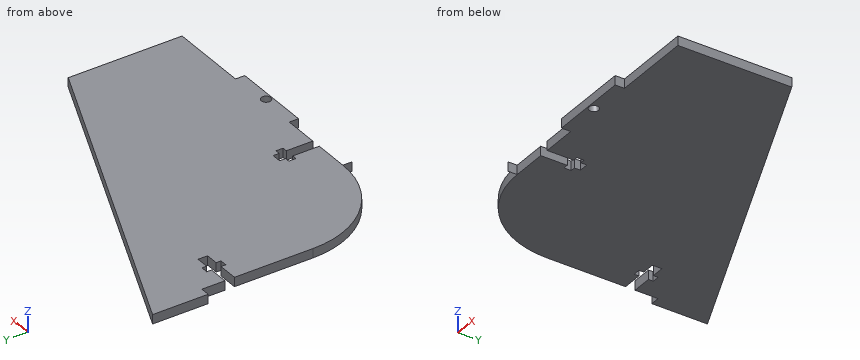
from build123d import *

# Parameters (mm, degrees)
BOSS_EXTRUDE1_DEPTH     = 2.9718
SKETCH3_W               = 2.9718
SKETCH3_H               = 17.78
CUT_EXTRUDE4_DEPTH      = 2.9718
CUT_EXTRUDE4_DEPTH_BACK = 3.9718
SKETCH4_R               = 1.524
CUT_EXTRUDE5_DEPTH      = 2.9718
CUT_EXTRUDE6_DEPTH      = 2.9718
CUT_EXTRUDE7_DEPTH      = 1
CUT_EXTRUDE7_DEPTH_BACK = 2.9718


with BuildPart() as part:
    # Sketch1 → Boss-Extrude1 (new body)
    with BuildSketch(Plane.XY):
        with BuildLine():
            Line((0, 0), (-76.2, 0))
            ThreePointArc((-76.2, 0), (-99.068034345, 9.472249971), (-108.540284316, 32.340284316))
            Line((-108.540284316, 32.340284316), (-108.540284316, 85.680284316))
            Line((-108.540284316, 85.680284316), (0, 39.416788246))
            Line((0, 39.416788246), (0, 0))
        make_face()
    extrude(amount=BOSS_EXTRUDE1_DEPTH)

    # Sketch3 → Cut-Extrude4 (cut, two sides)
    with BuildSketch(Plane.XY.offset(2.9718)) as cut_extrude4_sk:
        Polygon((-25.342092582, 2.9718), (-25.349200788, 0), (0, 0), (0, 2.9718), align=None)
        with BuildLine():
            Line((-76.2, 2.9718), (-76.202051529, 6.5e-08))
            ThreePointArc((-76.202051529, 6.5e-08), (-76.201025765, 1.6e-08), (-76.2, 0))
            Line((-76.2, 0), (-50.8, 0))
            Line((-50.8, 0), (-50.8, 2.9718))
            Line((-50.8, 2.9718), (-76.2, 2.9718))
        make_face()
        with Locations((-107.054384316, 59.010284316)):
            Rectangle(SKETCH3_W, SKETCH3_H)
    extrude(amount=CUT_EXTRUDE4_DEPTH, mode=Mode.SUBTRACT)
    extrude(cut_extrude4_sk.sketch, amount=-CUT_EXTRUDE4_DEPTH_BACK, mode=Mode.SUBTRACT)

    # Sketch4 → Cut-Extrude5 (cut)
    with BuildSketch(Plane.XY.offset(2.9718)):
        with Locations((-38.074600394, 1.794277041)):
            Circle(SKETCH4_R)
    extrude(amount=-CUT_EXTRUDE5_DEPTH, mode=Mode.SUBTRACT)

    # Sketch5 → Cut-Extrude6 (cut)
    with BuildSketch(Plane.XY.offset(2.9718)):
        Polygon((-105.568484316, 60.534284316), (-105.568484316, 59.010284316), (-92.868484316, 59.010284316), (-92.868484316, 60.534284316), (-96.932484316, 60.534284316), (-96.932484316, 62.058284316), (-99.218484316, 62.058284316), (-99.218484316, 60.534284316), align=None)
        Polygon((-92.868484316, 59.010284316), (-105.568484316, 59.010284316), (-105.568484316, 57.486284316), (-99.218484316, 57.486284316), (-99.218484316, 55.962284316), (-96.932484316, 55.962284316), (-96.932484316, 57.486284316), (-92.868484316, 57.486284316), align=None)
        Polygon((-65.024, 2.9718), (-63.5, 2.9718), (-63.5, 15.6718), (-65.024, 15.6718), (-65.024, 13.745923506), (-66.548, 13.745923506), (-66.548, 11.459923506), (-65.024, 11.459923506), align=None)
        Polygon((-63.5, 15.6718), (-63.5, 2.9718), (-61.976, 2.9718), (-61.976, 11.459923506), (-60.452, 11.459923506), (-60.452, 13.745923506), (-61.976, 13.745923506), (-61.976, 15.6718), align=None)
    extrude(amount=-CUT_EXTRUDE6_DEPTH, mode=Mode.SUBTRACT)

    # Sketch6 → Cut-Extrude7 (cut, two sides)
    with BuildSketch(Plane.XY.offset(2.9718)) as cut_extrude7_sk:
        with BuildLine():
            ThreePointArc((-105.568484316, 32.340284316), (-96.967313076, 11.574288587), (-76.201863011, 2.971800059))
            Line((-76.201863011, 2.971800059), (-76.202051529, 6.5e-08))
            ThreePointArc((-76.202051529, 6.5e-08), (-99.068759659, 9.472975307), (-108.540284316, 32.340284316))
            Line((-108.540284316, 32.340284316), (-108.540284316, 50.120284316))
            Line((-108.540284316, 50.120284316), (-105.568484316, 50.120284316))
            Line((-105.568484316, 50.120284316), (-105.568484316, 32.340284316))
        make_face()
    extrude(amount=CUT_EXTRUDE7_DEPTH, mode=Mode.SUBTRACT)
    extrude(cut_extrude7_sk.sketch, amount=-CUT_EXTRUDE7_DEPTH_BACK, mode=Mode.SUBTRACT)


solid = part.part
The model under review builds one solid part; all positions refer to its coordinate system, in mm. Round coordinates to 2 decimals unless told otherwise and drop trailing zeros. Write each loop counter-clockwise with the first axis right and the second up, starting at its lowest first coordinate (ties: lowest second). Pieces come first, ordered by that corner, then holes. Notation, with made-up numbers: (22, 5) - (63, 5) arc R13 cw to (63, 26) - close; hole circle Ø7 at (84.25, 49). An arc over 180 degrees is marked (long way). One line per item, written item: value. Start each with the question number.
1. Clearance check with flat-ended pins moving along their axes: P1, Ø1, axis at x = -91, z = 2, coming from the +Y side; P2, Ø0.8, axis at x = -61.5, z = 1, coming from the -Y side; P3, Ø1.5, axis at y = 5, z = 2, coming from the -X side; P4, Ø0.6, axis at y = 14.5, z = 1, coming from the +X side. State where each tip first meets the part, or that it passes through.
2. Consider section A-A on y = 17. Write out the cut boundary in (x, z), and give its area (3 significant figures).
3. Consider section B-B on x = -23. Write out the cut boundary in (y, z).
4. To check wall thickness, follow L1, parallel to Y at x = -100, z = 0.85; L2, parallel to X at y = 32, z = 2.6; L3, parallel to Y at x = -101, z = 2.4. State the ranges of each line that lie inside material, in increasing order. Write a range as from..to.
Checks:
1. P1: stops at y = 78.42
1. P2: stops at y = 2.97
1. P3: stops at x = -88.67
1. P4: stops at x = 0
2. outline: (-101.24, 0) - (0, 0) - (0, 2.97) - (-101.24, 2.97) - close
2. area: 301 mm^2
3. outline: (2.97, 0) - (49.22, 0) - (49.22, 2.97) - (2.97, 2.97) - close
4. L1: y = 15.13..57.49, 60.53..82.04
4. L2: x = -105.57..0
4. L3: y = 16.61..57.49, 60.53..82.47
